from build123d import *

# Parameters (mm, degrees)
BOSS_EXTRUDE1_DEPTH  = 5.8
BOSS_EXTRUDE2_DEPTH  = 3.6
M3_CLEARANCE_HOLE1_D = 3.4
CUT_EXTRUDE1_DEPTH   = 4
FILLET1_R            = 0.5


with BuildPart() as part:
    # Sketch1 → Boss-Extrude1 (new body)
    with BuildSketch(Plane(origin=(0, 0, 0), x_dir=(1, 0, 0), z_dir=(0, 1, 0))):
        with BuildLine():
            Line((-18.5, 0), (18.5, 0))
            Line((18.5, 0), (18.5, 10))
            Line((18.5, 10), (6.5, 10))
            ThreePointArc((6.5, 10), (0, 3.5), (-6.5, 10))
            Line((-6.5, 10), (-18.5, 10))
            Line((-18.5, 10), (-18.5, 0))
        make_face()
    extrude(amount=BOSS_EXTRUDE1_DEPTH)

    # Sketch7 → Boss-Extrude2 (add)
    with BuildSketch(Plane(origin=(0, 5.8, 0), x_dir=(1, 0, 0), z_dir=(0, 1, 0))):
        with BuildLine():
            Line((-18.5, 10), (-18.5, 0))
            Line((-18.5, 0), (18.5, 0))
            Line((18.5, 0), (18.5, 10))
            Line((18.5, 10), (8.5, 10))
            ThreePointArc((8.5, 10), (0, 1.5), (-8.5, 10))
            Line((-8.5, 10), (-18.5, 10))
        make_face()
    extrude(amount=BOSS_EXTRUDE2_DEPTH)

    # M3 Clearance Hole1 (through all)
    with Locations(Plane.XY):
        with Locations((-13.5, 4.7), (13.5, 4.7)):
            Hole(M3_CLEARANCE_HOLE1_D / 2)

    # Sketch5 → Cut-Extrude1 (cut)
    with BuildSketch(Plane.XY):
        with BuildLine():
            Line((-11.395542808, 9.4), (-18.5, 9.4))
            Line((-18.5, 9.4), (-18.5, 0))
            Line((-18.5, 0), (-11.395542808, 0))
            ThreePointArc((-11.395542808, 0), (-7.140159789, 4.7), (-11.395542808, 9.4))
        make_face()
        with BuildLine():
            Line((18.5, 0), (11.395542808, 0))
            ThreePointArc((11.395542808, 0), (7.140159789, 4.7), (11.395542808, 9.4))
            Line((11.395542808, 9.4), (18.5, 9.4))
            Line((18.5, 9.4), (18.5, 0))
        make_face()
    extrude(amount=-CUT_EXTRUDE1_DEPTH, mode=Mode.SUBTRACT)

    # Fillet1
    fillet1_edges = [part.edges().sort_by_distance(p)[0] for p in [
        (-11.395542808, 9.4, -2),
        (-11.395542808, 0, -2),
        (11.395542808, 0, -2),
        (11.395542808, 9.4, -2),
    ]]
    fillet(fillet1_edges, radius=FILLET1_R)


solid = part.part
Input: part model. Units: mm. Frame: model coordinates. A direction names the side the tool comes from. Round coordinates to 2 decimals unless told otherwise and drop trailing zeros. Loops run counter-clockwise (first coordinate to the right, second up) from the corner with the lowest first, then second, coordinate; pieces in that order, holes last. Notation, with made-up numbers: M 20.5,-15.75 L 28.5,-15.75 A16 ccw 28.5,10.25 Z; hole C -21.5,-2 d10. An arc over 180 degrees is marked long. Answer as CSV lines item,"result". Start each with the question number.
(1) First-contact query: pin 1 (1.5 mm diameter, centred on x = -4, y = 1, fed in from -Z); pin 2 (3 mm diameter, centred on x = -13.5, y = 5, fed in from +Z); pin 3 (4 mm diameter, centred on x = -2, y = 1.5, fed in from -Z). Flat tips, straight axial feed; report the tip coordinate or a pass-through.
(2) Line query: line 1 (Y direction, x = -13.5, z = -5.65); line 2 (X direction, y = 5.25, z = -8); line 3 (Z direction, x = -14.5, y = 6.25). Output: solid intervals per line, ascending. Write a range as [from, to].
(3) Section C-C, the plane z = -6.5. Output: boundary loops of the cut face in (x, y), plus the area to 3 significant figures.
(4) Section B-B, the plane y = 4.7. Output: boundary loops of the cut face in (x, z), plus the area to 3 significant figures.
(5) Draft query along Y for faces 5 (the flat face through (-1, 5.8, -3)), 6 (the flat face through (-18.5, 5, -7)), 7 (the cylindrical face through (9.23, 9.06, -2.03)). Return one class per face: released by +Y, released by -Y, zero draft, split by the parting line, or undercut.
(6) Reachability of faces 1 (the cylindrical face through (0.187, 7.575, -1.502)), 2 (the cylindrical face through (7.14, 4.64, -1.97)), 3 (the cylindrical face through (-14.414, 6.133, -7.042)), 4 (the cylindrical face through (-9.23, 9.06, -2.03)) from +Z, -Z, +X, -X, +Y, -Y: full face, straight path, thin tool, end or side. Return the list, or none.
(7) Section D-D, the plane y = 0.5. Output: boundary loops of the cut face in (x, z).
(8) Section A-A, the plane x = -13.5. Output: boundary loops of the cut face in (y, z).
Values found:
1,pin 1,"stops at z = -5.56"
1,pin 2,"stops at z = -4"
1,pin 3,"stops at z = -4.88"
2,line 1,"y = [0, 3], [6.4, 9.4]"
2,line 2,"x = [-18.5, -15.11], [-11.89, -6.18], [6.18, 11.89], [15.11, 18.5]"
2,line 3,"z = [-10, -4]"
3,outline,"M -18.5,0 L -5.48,0 L -5.48,5.8 L -7.75,5.8 L -7.75,9.4 L -18.5,9.4 Z; M 5.48,0 L 18.5,0 L 18.5,9.4 L 7.75,9.4 L 7.75,5.8 L 5.48,5.8 Z; hole C -13.5,4.7 d3.4; hole C 13.5,4.7 d3.4"
3,area,"210 mm²"
4,outline,"M -18.5,-10 L -15.2,-10 L -15.2,-4 L -18.5,-4 Z; M -11.8,-10 L -6.5,-10 A6.5 cw 6.5,-10 L 11.8,-10 L 11.8,-4 L 7.14,-4 L 7.14,0 L -7.14,0 L -7.14,-4 L -11.8,-4 Z; M 15.2,-10 L 18.5,-10 L 18.5,-4 L 15.2,-4 Z"
4,area,"172 mm²"
5,face 5,"released by +Y"
5,face 6,"zero draft"
5,face 7,"undercut"
6,face 1,"-Z, +Y"
6,face 2,"+Z, +X"
6,face 3,"+Z, -Z"
6,face 4,"+Z, -X"
7,outline,"M -18.5,-10 L -6.5,-10 A6.5 cw 6.5,-10 L 18.5,-10 L 18.5,-4 L 9.26,-4 L 9.26,0 L -9.26,0 L -9.26,-4 L -18.5,-4 Z"
8,outline,"M 0,-10 L 3,-10 L 3,-4 L 0,-4 Z; M 6.4,-10 L 9.4,-10 L 9.4,-4 L 6.4,-4 Z"
